Answer from the drawing. Dimensions are ordinates in mm from the lowest x, y and z of the part. A direction names the side the tool comes from. Round coordinates to 2 decimals unless told otherwise and drop trailing zeros. Write each loop counter-clockwise with the first axis right and the second up, starting at its lowest first coordinate (ties: lowest second). Pieces come first, ordered by that corner, then holes. Notation, with made-up numbers: (-12, 48.25) - (0, 48.25) arc R28 cw to (0, 68.25) - close; hole circle Ø6 at (-35.5, -34.5). An arc over 180 degrees is marked (long way). Use a Markdown table: item, result. Add a question column.
1) A cutting plane is placed at A-A (x = 4.5). Give the vertices of the cut face in (y, z) (1 decimal).
2) A cutting plane is placed at B-B (z = 8.5). Give the vertices of the cut face in (x, y), then the cut area to 3 significant figures.
3) This flat-tipped pin is pushed along its axis until it touches: P1, Ø3, axis at x = 8.5, y = 7.5, coming from the -Z side. Where does it stop, or does it pass through?
4) Find the intervals of material crossed by probe 1 along Z at (x, y) = (7.5, 4.25); probe 2 along Z at (x, y) = (3.25, 6) (1 decimal); probe 3 along Z at (x, y) = (3.75, 3.5), in increasing order. Write a range as from..to.
5) A tool of negligible diameter and unlimited length cuts with its end or side. For the marked faces 4 and 5, from which of +Z, -Z, +X, -X, +Y, -Y can it reach the whole face along a straight path? Write none if from no direction.
6) A cutting plane is placed at C-C (x = 8). Give the vertices of the cut face in (y, z).
7) Determine the mould class of the marked faces 1, 2 and 3 for opening direction Z: +Z half, -Z half, draft (parallel to the pull), parting line (faces both ways), or undercut.
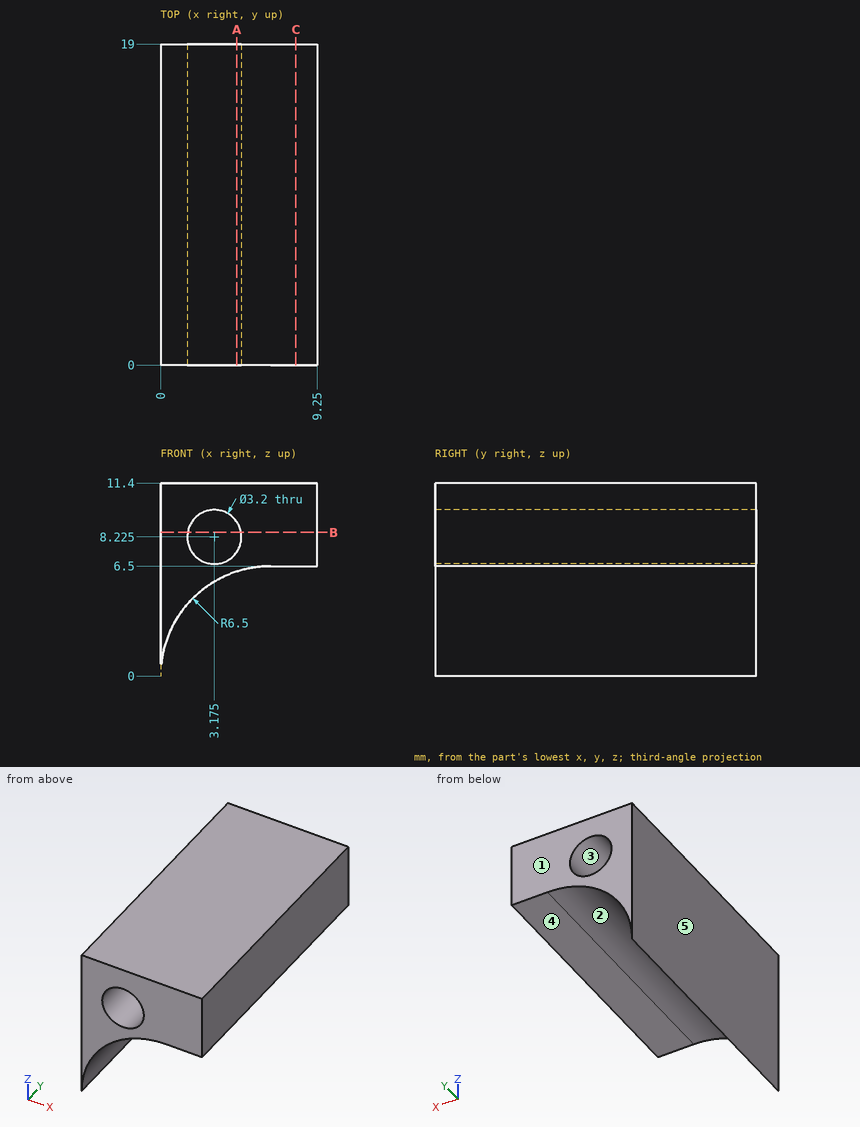
Entries:
| question | item | result |
|---|---|---|
| 1 | outline | (0, 6.2) - (19, 6.2) - (19, 7.3) - (0, 7.3) - close; (0, 9.1) - (19, 9.1) - (19, 11.4) - (0, 11.4) - close |
| 2 | outline | (0, 0) - (1.6, 0) - (1.6, 19) - (0, 19) - close; (4.75, 0) - (9.25, 0) - (9.25, 19) - (4.75, 19) - close |
| 2 | area | 116 mm² |
| 3 | P1 | stops at z = 6.5 |
| 4 | probe 1 | z = 6.5..11.4 |
| 4 | probe 2 | z = 5.6..6.6, 9.8..11.4 |
| 4 | probe 3 | z = 5.89..6.73, 9.72..11.4 |
| 5 | face 4 | -Z, +X, +Y, -Y |
| 5 | face 5 | +Z, -Z, -X, +Y, -Y |
| 6 | outline | (0, 6.5) - (19, 6.5) - (19, 11.4) - (0, 11.4) - close |
| 7 | face 1 | draft |
| 7 | face 2 | -Z half |
| 7 | face 3 | undercut |
